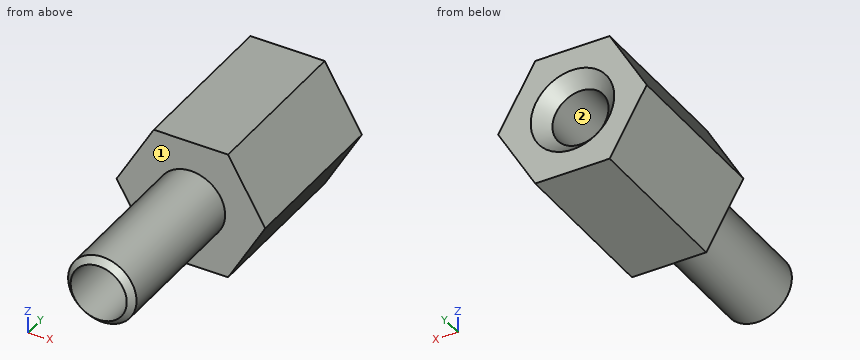
from build123d import *

# Parameters (mm, degrees)
BOSS_EXTRUDE1_DEPTH                = 6
SKETCH2_W                          = 1.25
SKETCH2_H                          = 6
TAP_DRILL_FOR_M2_5X0_45_TAP1_D     = 2.05
TAP_DRILL_FOR_M2_5X0_45_TAP1_DEPTH = 19
CHAMFER1_SIZE                      = 0.5


with BuildPart() as part:
    # Sketch1 → Boss-Extrude1 (new body)
    with BuildSketch(Plane(origin=(0, 6, 0), x_dir=(1, 0, 0), z_dir=(0, 1, 0))):
        Polygon((1.356773133, -2.35), (2.713546265, 0), (1.356773133, 2.35), (-1.356773133, 2.35), (-2.713546265, 0), (-1.356773133, -2.35), align=None)
    extrude(amount=-BOSS_EXTRUDE1_DEPTH)

    # Sketch2 → Revolve1 (revolve)
    with BuildSketch(Plane(origin=(0, 0, 0), x_dir=(-1, 0, 0), z_dir=(0, 0, -1)), mode=Mode.PRIVATE) as revolve1_sk:
        with Locations((-0.625, -3)):
            Rectangle(SKETCH2_W, SKETCH2_H)
    revolve(revolve1_sk.sketch.rotate(Axis((0, -6, 0), (0, 1, 0)), 270), axis=Axis((0, -6, 0), (0, 1, 0)))

    # Tap Drill for M2.5x0.45 Tap1
    with Locations(Plane(origin=(0, 6, 0), x_dir=(1, 0, 0), z_dir=(0, 1, 0))):
        with Locations((0, 0)):
            Hole(TAP_DRILL_FOR_M2_5X0_45_TAP1_D / 2, depth=TAP_DRILL_FOR_M2_5X0_45_TAP1_DEPTH)

    # Chamfer1
    # the kernel refuses this chamfer: 0.5 mm, written as the material it takes off along each edge
    with BuildSketch(Plane(origin=(0, -6, 0), x_dir=(0, 0, 1), z_dir=(-1, 0, 0))) as chamfer1_piece_1:
        Polygon((1.25, CHAMFER1_SIZE), (1.25 - CHAMFER1_SIZE, 0), (1.25, 0), align=None)
    revolve(axis=Axis((0, -6, 0), (0, 1, 0)), mode=Mode.SUBTRACT)
    with BuildSketch(Plane(origin=(0, 6, 0), x_dir=(-1, 0, 0), z_dir=(0, 0, 1))) as chamfer1_piece_2:
        Polygon((1.025 + CHAMFER1_SIZE, 0), (1.025, CHAMFER1_SIZE), (1.025, 0), align=None)
    revolve(axis=Axis((0, 6, 0), (0, -1, 0)), mode=Mode.SUBTRACT)


solid = part.part
The listing builds one solid part. Answer for the finished solid, in the listing's coordinates (mm). Face numbers are marked on the shaded views. A direction names the side the tool comes from. Coordinates: 2 decimals unless noted, no trailing zeros. Write each loop counter-clockwise with the first axis right and the second up, starting at its lowest first coordinate (ties: lowest second). Pieces come first, ordered by that corner, then holes. Notation, with made-up numbers: (-35, 10) - (-19, 10) arc R23 cw to (-19, 18) - close; hole circle Ø5 at (24.5, 81.25). An arc over 180 degrees is marked (long way). Answer as CSV lines item,"result".
1. Given P1, Ø2, axis at x = -2, y = -3, coming from the -Z side; P2, Ø2, axis at y = -2.5, z = -1, coming from the +X side, each flat-ended and moving along its own axis, determine where each tip first touches the part or whether it passes through.
Computed values:
P1,"stops at z = -0.75"
P2,"stops at x = 1.25"
2. Find section C-C (y = -2). Give the vertices of the cut face in (x, z) (3 decimals), plus the area to 3 significant figures.
Computed values:
outline,"circle Ø2.5 at (0, 0); hole circle Ø2.05 at (0, 0)"
area,"1.61 mm²"
3. Find section B-B (y = 3.5). Give the vertices of the cut face in (x, z) (3 decimals).
Computed values:
outline,"(-2.714, 0) - (-1.357, -2.35) - (1.357, -2.35) - (2.714, 0) - (1.357, 2.35) - (-1.357, 2.35) - close; hole circle Ø2.05 at (0, 0)"
4. Straight lines are drawn through the part: line 1 (X direction, y = -2, z = 0) (3 decimals); line 2 (Z direction, x = 0, y = 2.5) (3 decimals); line 3 (Y direction, x = -0.95, z = 1.9). For each, find the intervals that lie inside material, in ascending order. Write a range as [from, to].
Computed values:
line 1,"x = [-1.25, -1.025], [1.025, 1.25]"
line 2,"z = [-2.35, -1.025], [1.025, 2.35]"
line 3,"y = [0, 6]"
5. A tool of negligible diameter and unlimited length cuts with its end or side. For the marked faces 1 and 2, from which of +Z, -Z, +X, -X, +Y, -Y can it reach the whole face along a straight path? Write none if from no direction.
Computed values:
face 1,"-Y"
face 2,"+Y, -Y"
6. Find section D-D (x = 2.15). Give the vertices of the cut face in (y, z).
Computed values:
outline,"(0, -0.98) - (6, -0.98) - (6, 0.98) - (0, 0.98) - close"
7. Find section A-A (x = 0). Give the vertices of the cut face in (y, z) (3 decimals), plus the area to 3 significant figures.
Computed values:
outline,"(-5.725, -1.025) - (-5.5, -1.25) - (0, -1.25) - (0, -2.35) - (6, -2.35) - (6, -1.525) - (5.5, -1.025) - close; (-5.725, 1.025) - (5.5, 1.025) - (6, 1.525) - (6, 2.35) - (0, 2.35) - (0, 1.25) - (-5.5, 1.25) - close"
area,"18.2 mm²"
